Check sheet for the modelled part. Datum: model origin and axes. Units: mm. A direction names the side the tool comes from. Round coordinates to 2 decimals unless told otherwise and drop trailing zeros. Write each loop counter-clockwise with the first axis right and the second up, starting at its lowest first coordinate (ties: lowest second). Pieces come first, ordered by that corner, then holes. Notation, with made-up numbers: M -26.75,72 L 32.25,72 A30 cw 32.25,94 Z; hole C 47,-26 d3. An arc over 180 degrees is marked long. Put each result on its own line as item: value.
```python
from build123d import *

# Parameters (mm, degrees)
SKETCH1_R           = 38.1
BOSS_EXTRUDE1_DEPTH = 41.275
SKETCH2_R           = 15.875
BOSS_EXTRUDE2_DEPTH = 127
SKETCH3_R           = 38.1
BOSS_EXTRUDE3_DEPTH = 6.35
BOSS_EXTRUDE4_DEPTH = 165.1
CUT_EXTRUDE1_REACH  = 370.861


with BuildPart() as part:
    # Sketch1 → Boss-Extrude1 (new, symmetric)
    with BuildSketch(Plane(origin=(0, 0, 0), x_dir=(1, 0, 0), z_dir=(0, 1, 0))):
        with Locations(Location((0, 0, 0), (0, 0, 270))):
            Circle(SKETCH1_R)
    extrude(amount=BOSS_EXTRUDE1_DEPTH, both=True)

    # Sketch2 → Boss-Extrude2 (add)
    with BuildSketch(Plane.XZ.offset(41.275)):
        with Locations(Location((0, 0, 0), (0, 0, 270))):
            Circle(SKETCH2_R)
    extrude(amount=BOSS_EXTRUDE2_DEPTH)

    # Sketch3 → Boss-Extrude3 (add)
    with BuildSketch(Plane.XZ.offset(168.275)):
        with Locations(Location((0, 0, 0), (0, 0, 90))):
            Circle(SKETCH3_R)
    extrude(amount=BOSS_EXTRUDE3_DEPTH)

    # Sketch4 → Boss-Extrude4 (add)
    with BuildSketch(Plane.XZ.offset(174.625)):
        with BuildLine():
            Line((-50.8, 38.1), (-50.8, 101.6))
            Line((-50.8, 101.6), (50.8, 101.6))
            Line((50.8, 101.6), (50.8, 38.1))
            ThreePointArc((50.8, 38.1), (0, -12.7), (-50.8, 38.1))
        make_face()
    extrude(amount=BOSS_EXTRUDE4_DEPTH)

    # Cut-Extrude1: up to this face of the body (flat: up to its plane)
    cut_extrude1_end = Plane(part.part.faces().sort_by_distance((-50.8, -257.175, 69.85))[0])
    # Sketch5 → Cut-Extrude1 (cut, up to the picked face)
    with BuildSketch(Plane(origin=(50.8, 0, 0), x_dir=(0, 0, -1), z_dir=(1, 0, 0)), mode=Mode.PRIVATE) as cut_extrude1_sk1:
        Polygon((-38.1, -174.625), (-101.6, -174.625), (-101.6, -250.825), align=None)
    cut_extrude1_tool1 = split(extrude(cut_extrude1_sk1.sketch, amount=-CUT_EXTRUDE1_REACH, mode=Mode.PRIVATE), bisect_by=cut_extrude1_end, keep=Keep.BOTH, mode=Mode.PRIVATE)
    add(cut_extrude1_tool1.solids().sort_by(Axis((50.8, -200.025, 80.433333), (-1, 0, 0)))[0], mode=Mode.SUBTRACT)

    # Sketch6 → Revolve1 (revolve)
    with BuildSketch(Plane.XY, mode=Mode.PRIVATE) as revolve1_sk:
        Polygon((0, 41.275), (50.8, 41.275), (38.1, 149.225), (38.1, 168.275), (0, 168.275), align=None)
    revolve(revolve1_sk.sketch.rotate(Axis((0, 168.275, 0), (0, -1, 0)), 180), axis=Axis((0, 168.275, 0), (0, -1, 0)))


solid = part.part
```
1. Access from +Z, -Z, +X, -X, +Y, -Y to the whole of each face (thin tool, end or side, straight path). Record for faces 4 (the cylindrical face through (1.117, -256.019, -12.688)), 5 (the flat face through (-1, -168.275, 16)), 6 (the flat face through (35, -174.625, 28)), 7 (the cylindrical face through (8.259, 158.883, 37.194)), 8 (the flat face through (-37, -174.625, 26)).
Computed values:
face 4: -Z, -Y
face 5: none
face 6: +Z, +X
face 7: +Y
face 8: +Z, -X
2. Depth check by flat-ended pin: pin 1 Ø5 at (y, z) = (89, -7) entering from -X; pin 2 Ø4 at (x, y) = (33.5, 114) entering from -Z; pin 3 Ø2 at (y, z) = (23, 7) entering from -X. Enter the tip coordinate at first touch or a pass-through.
Computed values:
pin 1: stops at x = -45.09
pin 2: stops at z = -28.18
pin 3: stops at x = -37.62
3. Cross-section at A-A (y = -46). Enter the section's corners in (x, z) (3 decimals), then the cut area to 3 significant figures.
Computed values:
outline: C 0,0 d31.75
area: 792 mm2
4. Cross-section at B-B (y = -230). Enter the section's corners in (x, z), then the cut area to 3 significant figures.
Computed values:
outline: M -50.8,38.1 A50.8 ccw 50.8,38.1 L 50.8,84.25 L -50.8,84.25 Z
area: 8,740 mm2
5. Release check for a two-part mould opening along Y. For faces 1 (the conical face through (35.2, 96, 27)), 2 (the cylindrical face through (-23.183, 0.578, -30.235)), 3 (the flat face through (50.8, -274, 70)) record: +Y half, -Y half, draft (parallel to the pull), parting line (faces both ways), or undercut.
Computed values:
face 1: +Y half
face 2: undercut
face 3: draft
6. Scan lines: probe 1 along Y at (x, z) = (-14, -22) (3 decimals); probe 2 along Z at (x, y) = (33, 94.5); probe 3 along X at (y, z) = (57, 29). Record each from-to range of solid material in increasing order.
Computed values:
probe 1: y = -174.625 to -168.275, -41.275 to 168.275
probe 2: z = -29.91 to 29.91
probe 3: x = -39.43 to 39.43
